CAD build for the part. Positions are in the model's coordinates, mm. A direction names the side the tool comes from. Round coordinates to 2 decimals unless told otherwise and drop trailing zeros. Order: outer loops, then holes, each group sorted by start corner. A loop starts at its lowest first (then second) coordinate and runs counter-clockwise, first axis right, second up. Notation, with made-up numbers: M 21,65.25 L 60,65.25 A23 cw 60,75.25 Z; hole C 46.25,-30 d6. An arc over 180 degrees is marked long. Put each result on its own line as item: value.
```python
from build123d import *
from OCP.BRepFilletAPI import BRepFilletAPI_MakeChamfer

# Parameters (mm, degrees)
TOPSKETCH1_R                         = 1
TOPBOSS_EXTRUDE1_DEPTH               = 2
RAILCLAMPBOSS_EXTRUDE2_DEPTH         = 10
RAILSCREWSIDE1HOLECUT_EXTRUDE1_REACH = 42.596
RAILSCREWSIDE1HOLESKETCH3_R          = 1.75
RAILSCREWSIDE2HOLECUT_EXTRUDE2_REACH = 42.596
RAILSCREWSIDE2HOLESKETCH4_R          = 1.25
FILLET1_R                            = 10
CHAMFER2_SIZE                        = 10
CHAMFER2_SIZE2                       = 12


with BuildPart() as part:
    # TopSketch1 → TopBoss-Extrude1 (new body)
    with BuildSketch(Plane(origin=(0, 0, 0), x_dir=(1, 0, 0), z_dir=(0, 1, 0))):
        Polygon((0, 0), (29, 0), (29, 37.5), (0, 37.5), (0, 22.75), (21, 22.75), (21, 14.75), (0, 14.75), align=None)
        with Locations(Location((8.5, 32.5, 0), (0, 0, 270))):
            Circle(TOPSKETCH1_R, mode=Mode.SUBTRACT)
        with Locations(Location((8.5, 5, 0), (0, 0, 270))):
            Circle(TOPSKETCH1_R, mode=Mode.SUBTRACT)
    extrude(amount=TOPBOSS_EXTRUDE1_DEPTH)

    # RailClampSketch2 → RailClampBoss-Extrude2 (add)
    with BuildSketch(Plane(origin=(0, 2, 0), x_dir=(1, 0, 0), z_dir=(0, 1, 0))):
        Polygon((0, 37.5), (0, 22.75), (21, 22.75), (21, 14.75), (0, 14.75), (0, 0), (2, 0), (2, 11.75), (21, 11.75), (21, 0), (23, 0), (23, 37.5), (21, 37.5), (21, 25.75), (2, 25.75), (2, 37.5), align=None)
    extrude(amount=RAILCLAMPBOSS_EXTRUDE2_DEPTH)

    # RailScrewSide1HoleSketch3 → RailScrewSide1HoleCut-Extrude1 (cut, up to next)
    with BuildSketch(Plane.XY.offset(-11.75), mode=Mode.PRIVATE) as railscrewside1holecut_extrude1_sk1:
        with Locations((7.425, 6)):
            Circle(RAILSCREWSIDE1HOLESKETCH3_R)
    railscrewside1holecut_extrude1_tool1 = extrude(railscrewside1holecut_extrude1_sk1.sketch, amount=-RAILSCREWSIDE1HOLECUT_EXTRUDE1_REACH, mode=Mode.PRIVATE) & part.part
    add(railscrewside1holecut_extrude1_tool1.solids().sort_by_distance((7.425, 6, -11.75))[0], mode=Mode.SUBTRACT)

    # RailScrewSide2HoleSketch4 → RailScrewSide2HoleCut-Extrude2 (cut, up to next)
    with BuildSketch(Plane(origin=(0, 0, -25.75), x_dir=(-1, 0, 0), z_dir=(0, 0, -1)), mode=Mode.PRIVATE) as railscrewside2holecut_extrude2_sk1:
        with Locations((-7.425, 6)):
            Circle(RAILSCREWSIDE2HOLESKETCH4_R)
    railscrewside2holecut_extrude2_tool1 = extrude(railscrewside2holecut_extrude2_sk1.sketch, amount=-RAILSCREWSIDE2HOLECUT_EXTRUDE2_REACH, mode=Mode.PRIVATE) & part.part
    add(railscrewside2holecut_extrude2_tool1.solids().sort_by_distance((7.425, 6, -25.75))[0], mode=Mode.SUBTRACT)

    # Fillet1
    fillet1_edges = [part.edges().sort_by_distance(p)[0] for p in [
        (0, 6, 0),
        (0, 6, -37.5),
    ]]
    fillet(fillet1_edges, radius=FILLET1_R)

    # Chamfer2: one chamfer whose edges measure the first distance from different faces: ONE call of the kernel's chamfer builder (chamfer() names one face for all edges)
    chamfer2_edges_1 = [part.edges().sort_by_distance(p)[0] for p in [
        (22, 12, -37.5),
    ]]
    chamfer2_side_1 = [part.faces().sort_by_distance(p)[0] for p in [
        (15.5, 1.775277949, -37.5),
    ]]
    chamfer2_edges_2 = [part.edges().sort_by_distance(p)[0] for p in [
        (22, 12, 0),
    ]]
    chamfer2_side_2 = [part.faces().sort_by_distance(p)[0] for p in [
        (15.5, 1.775277949, 0),
    ]]
    chamfer2 = BRepFilletAPI_MakeChamfer(part.part.solid().wrapped)
    for e in chamfer2_edges_1:
        chamfer2.Add(CHAMFER2_SIZE, CHAMFER2_SIZE2, e.wrapped, chamfer2_side_1[0].wrapped)  # the first distance lies on this face
    for e in chamfer2_edges_2:
        chamfer2.Add(CHAMFER2_SIZE, CHAMFER2_SIZE2, e.wrapped, chamfer2_side_2[0].wrapped)  # the first distance lies on this face
    add(Compound.cast(chamfer2.Shape()), mode=Mode.REPLACE)


solid = part.part
```
Item 1: Tool access for faces 4 (the flat face through (21, 6, -7)), 5 (the flat face through (2, 6, -29)), 6 (the cylindrical face through (6.036, 4.935, -13.229)), 7 (the flat face through (26, 2, -19)): list every direction of +Z, -Z, +X, -X, +Y, -Y with a clear straight run to the whole face (end or side of a thin tool).
Answers below:
face 4: +Z, +Y
face 5: -Z, +Y
face 6: +Z
face 7: +Z, -Z, +X, +Y
Item 2: Band-saw the part on D-D on z = -32. Give the cut face in (x, y).
Answers below:
outline: M 1.07,0 L 7.63,0 L 7.63,2 L 2,2 L 2,6.58 L 1.07,6.58 Z; M 9.37,0 L 29,0 L 29,2 L 23,2 L 23,6.58 L 21,6.58 L 21,2 L 9.37,2 Z
Item 3: Band-saw the part on B-B on y = 6. Give the cut face in (x, z) (3 decimals).
Answers below:
outline: M 0,-27.5 A10 ccw 1.458,-32.7 L 2,-32.7 L 2,-25.75 L 6.175,-25.75 L 6.175,-22.75 L 0,-22.75 Z; M 0,-14.75 L 5.675,-14.75 L 5.675,-11.75 L 2,-11.75 L 2,-4.8 L 1.458,-4.8 A10 ccw 0,-10 Z; M 8.675,-25.75 L 21,-25.75 L 21,-32.7 L 23,-32.7 L 23,-4.8 L 21,-4.8 L 21,-11.75 L 9.175,-11.75 L 9.175,-14.75 L 21,-14.75 L 21,-22.75 L 8.675,-22.75 Z
Item 4: Probe line 1 along Z through (x, y) = (10.5, 6.5); line 2 along X through (y, z) = (9.5, -27.5); line 3 along X through (y, z) = (8, -19). List the from-to ranges inside material, lowest first. Write a range as [from, to].
Answers below:
line 1: [-25.75, -22.75], [-14.75, -11.75]
line 2: [0, 2], [21, 23]
line 3: [21, 23]
Item 5: Band-saw the part on A-A on x = 12.75. Give the cut face in (y, z).
Answers below:
outline: M 0,-37.5 L 2,-37.5 L 2,-25.75 L 11.79,-25.75 L 12,-25.5 L 12,-22.75 L 0,-22.75 Z; M 0,-14.75 L 12,-14.75 L 12,-12 L 11.79,-11.75 L 2,-11.75 L 2,0 L 0,0 Z
Item 6: Band-saw the part on C-C on x = 8. State how many separate pieces and enclosed holes the cut face has, and give its area (3 significant figures).
Answers below:
separate pieces: 6
enclosed holes: 0
area: 94.6 mm²
Item 7: Mould opens along Z. For faces 1 (the flat face through (19, 1, 0)), 2 (the flat face through (11, 2, -32)), 3 (the flat face through (10, 6, -22.75)) say: pulls with the +Z half, pulls with the -Z half, needs draft (parallel to the pull), parting line crosses it, or undercut.
Answers below:
face 1: pulls with the +Z half
face 2: needs draft
face 3: undercut
Item 8: Pin check, flat tips, straight feed: P1, Ø1, axis at x = 10, y = 4, coming from the -Z side; P2, Ø1, axis at y = 10, z = -21, coming from the -X side; P3, Ø4.5, axis at x = 7.425, y = 6, coming from the +Z side. Stop position of each tip, or through.
Answers below:
P1: z = -25.75
P2: x = 21
P3: z = -11.75
